Verification items for the finished model (mm, model axes). A direction names the side the tool comes from. Coordinates: 2 decimals unless noted, no trailing zeros. Write each loop counter-clockwise with the first axis right and the second up, starting at its lowest first coordinate (ties: lowest second). Pieces come first, ordered by that corner, then holes. Notation, with made-up numbers: (11, 68.25) -> (26, 68.25) arc R36 cw to (26, 106.25) -> close; hole circle Ø7 at (-8.5, 20.5). An arc over 180 degrees is marked (long way). Use CSV: the item, a comma, the result in double quotes.
Autodesk Inventor part; units mm, degrees
ref_plane "YZ Plane" through (0, 0, 0) normal (1, 0, 0) x (0, 1, 0)
ref_plane "XZ Plane" through (0, 0, 0) normal (0, 1, 0) x (-1, 0, 0)
ref_plane "XY Plane" through (0, 0, 0) normal (0, 0, 1) x (1, 0, 0)
sketch "Sketch1" plane through (0, 0, 0) normal (0, 1, 0) x (-1, 0, 0)
  line L0 (0, 0) -> (170, 0)
  line L1 (170, 0) -> (170, -320)
  line L2 (170, -320) -> (0, -320)
  line L3 (0, -320) -> (0, 0)
  dimension "d0" = 170
  dimension "d1" = 320
extrude "Extrusion1" add sketch "Sketch1" along normal blind 14
sketch "Sketch2" plane through (0, 14, 0) normal (0, 1, 0) x (1, 0, 0)
  line L0 (0, 320) -> (-170, 320)
  circle A0 centre (-85, 245) radius 30
  point P0 (0, 0)
  dimension "d5" = 60
extrude "Extrusion2" cut sketch "Sketch2" against normal blind 4
sketch "Sketch3" plane through (-85, 10, -245) normal (0, 1, 0) x (1, 0, 0)
  circle A0 centre (0, 0) radius 23.5
  point P0 (85, -245)
  dimension "d8" = 47
extrude "Extrusion3" cut sketch "Sketch3" against normal blind 9
sketch "Sketch4" plane through (-85, 1, -245) normal (0, 1, 0) x (1, 0, 0)
  circle A0 centre (0, 0) radius 20
  point P0 (85, -245)
  dimension "d11" = 40
extrude "Extrusion4" cut sketch "Sketch4" against normal blind 1
sketch "Sketch5" plane through (0, 14, 0) normal (0, 1, 0) x (1, 0, 0)
  circle A0 centre (-85, 245) radius 30
  circle A1 centre (-85, 82.3) radius 12.5
  circle A2 centre (-100.5, 66.8) radius 1.6
  circle A3 centre (-100.5, 97.8) radius 1.6
  circle A4 centre (-69.5, 97.8) radius 1.6
  circle A5 centre (-69.5, 66.8) radius 1.6
  point P0 (0, 0)
  dimension "d15" = 25
  dimension "d22" = 3.2
  dimension "d23" = 3.2
  dimension "d24" = 3.2
  dimension "d25" = 3.2
extrude "Extrusion5" cut sketch "Sketch5" against normal blind 14 contours A1 | A2 | A3 | A4 | A5
sketch "Sketch6" plane through (0, 0, 0) normal (0, -1, 0) x (1, 0, 0)
  circle A0 centre (-85, -82.3) radius 12.5
  line L0 (-106.5, -103.8) -> (-63.5, -103.8)
  line L1 (-63.5, -103.8) -> (-63.5, -60.8)
  line L2 (-63.5, -60.8) -> (-106.5, -60.8)
  line L3 (-106.5, -60.8) -> (-106.5, -103.8)
  point P0 (0, 0)
  dimension "d30" = 43
  dimension "d31" = 43
extrude "Extrusion6" cut sketch "Sketch6" against normal blind 10
sketch "Sketch7" plane through (0, 0, 0) normal (0, -1, 0) x (1, 0, 0)
  circle A0 centre (-85, -82.3) radius 12.5
  line L0 (-85, -187.3) -> (-35, -187.3)
  line L1 (-35, -192.3) -> (-135, -192.3)
  line L2 (-135, -187.3) -> (-85, -187.3)
  arc A1 (-135, -187.3) -> (-135, -192.3) centre (-135, -189.8) ccw
  arc A2 (-35, -192.3) -> (-35, -187.3) centre (-35, -189.8) ccw
  point P0 (0, 0)
  dimension "d34" = 105
  dimension "d36" = 5
  dimension "d37" = 100
  dimension "d38" = 5
  dimension "d39" = 5
  dimension "d40" = 5
extrude "Extrusion7" cut sketch "Sketch7" against normal blind 14 contours L0 A2 L1 A1 L2
sketch "Sketch8" plane through (0, 14, 0) normal (0, 1, 0) x (1, 0, 0)
  point P0 (0, 0)
sketch "Sketch9" plane through (0, 14, 0) normal (0, 1, 0) x (1, 0, 0)
  line L0 (0, 320) -> (-170, 320)
  line L1 (0, 320) -> (0, 310)
  line L2 (0, 0) -> (0, 320)
  circle A0 centre (-10, 310) radius 1.6
  line L3 (-170, 310) -> (-160, 310) construction
  circle A1 centre (-160, 310) radius 1.6
  dimension "d43" = 10
  dimension "d45" = 3.2
  dimension "d48" = 3.2
extrude "Extrusion8" cut sketch "Sketch9" against normal blind 14
pattern_linear "Rectangular Pattern1" count 7 spacing 50 along (0, 0, 1) of "Extrusion8"
sketch "Sketch10" plane through (0, 14, 0) normal (0, 1, 0) x (1, 0, 0)
  circle A0 centre (-160, 310) radius 1.6
  circle A1 centre (-110, 310) radius 1.6
  circle A2 centre (-160, 10) radius 1.6
  circle A3 centre (-110, 10) radius 1.6
  point P0 (0, 0)
  dimension "d56" = 3.2
  dimension "d58" = 3.2
extrude "Extrusion9" cut sketch "Sketch10" against normal blind 14 contours A1 | A3
pattern_linear "Rectangular Pattern2" count 2 spacing 50 along (1, 0, 0) of "Extrusion9"
properties part number "b_base_cover_1"
1) Cross-section at C-C (y = 6.5). Give the number of separate pieces and of enclosed holes in the cut face, plus the area to 3 significant figures.
Return value:
separate pieces,"1"
enclosed holes,"21"
area,"50,200 mm2"
2) Cross-section at D-D (x = -132). Record the boundary of the cut face in (y, z), plus the area to 3 significant figures.
Return value:
outline,"(0, -320) -> (14, -320) -> (14, -192.3) -> (0, -192.3) -> close; (0, -187.3) -> (14, -187.3) -> (14, 0) -> (0, 0) -> close"
area,"4,410 mm2"
3) Set-up check for faces 1 (the flat face through (-84, 7, -192.3)), 2 (the cylindrical face through (-88.06, 5.56, -268.3)), 3 (the flat face through (-63.5, 5, -83)): record each of +Z, -Z, +X, -X, +Y, -Y from which the full face is reachable in a straight line by a thin tool's end or side.
Return value:
face 1,"+Y, -Y"
face 2,"+Y"
face 3,"-Y"
4) Scan lines: L1, parallel to Z at x = -110, y = 6.25; L2, parallel to X at y = 11.25, z = -310; L3, parallel to Z at x = -35, y = 4.25. Record each from-to range of solid material in increasing order.
Return value:
L1,"-320 to -311.6, -308.4 to -192.3, -187.3 to -11.6, -8.4 to 0"
L2,"-170 to -161.6, -158.4 to -111.6, -108.4 to -61.6, -58.4 to -11.6, -8.4 to 0"
L3,"-320 to -192.3, -187.3 to 0"
5) Cross-section at A-A (x = -85). Record the boundary of the cut face in (y, z), plus the area to 3 significant figures.
Return value:
outline,"(0, -320) -> (14, -320) -> (14, -275) -> (10, -275) -> (10, -268.5) -> (1, -268.5) -> (1, -265) -> (0, -265) -> close; (0, -225) -> (1, -225) -> (1, -221.5) -> (10, -221.5) -> (10, -215) -> (14, -215) -> (14, -192.3) -> (0, -192.3) -> close; (0, -187.3) -> (14, -187.3) -> (14, -94.8) -> (10, -94.8) -> (10, -103.8) -> (0, -103.8) -> close; (0, -60.8) -> (10, -60.8) -> (10, -69.8) -> (14, -69.8) -> (14, 0) -> (0, 0) -> close"
area,"3,180 mm2"
6) Mould release check, pull along Z, two halves, no side actions. Record for faces 4 (the flat face through (-84, 14, -158)), 5 (the cylindrical face through (-79.23, 12.03, -71.21)), 6 (the flat face through (-86, 7, -320)): released by +Z, released by -Z, zero draft, split by the parting line, or undercut.
Return value:
face 4,"zero draft"
face 5,"undercut"
face 6,"released by -Z"
7) Cross-section at B-B (z = -245). Record the boundary of the cut face in (x, y).
Return value:
outline,"(-170, 0) -> (-105, 0) -> (-105, 1) -> (-108.5, 1) -> (-108.5, 10) -> (-115, 10) -> (-115, 14) -> (-170, 14) -> close; (-65, 0) -> (0, 0) -> (0, 14) -> (-55, 14) -> (-55, 10) -> (-61.5, 10) -> (-61.5, 1) -> (-65, 1) -> close"
